from build123d import *

# Parameters (mm, degrees)
BOSS_EXTRUDE1_DEPTH = 80
SKETCH2_W           = 80
SKETCH2_H           = 80
BOSS_EXTRUDE2_DEPTH = 790


with BuildPart() as part:
    # Sketch1 → Boss-Extrude1 (new body)
    with BuildSketch(Plane.XY):
        Polygon((1040, 0), (0, 0), (0, -857.8), (80, -857.8), (80, -604.8), (960, -604.8), (960, -857.8), (1040, -857.8), align=None)
        Polygon((960, -524.8), (80, -524.8), (80, -361.670887123), (400.767069293, -80), (639.232930707, -80), (960, -361.670887123), align=None, mode=Mode.SUBTRACT)
        Polygon((729.892680056, -80), (960, -80), (960, -282.061056595), align=None, mode=Mode.SUBTRACT)
        Polygon((80, -282.061056595), (80, -80), (310.107319944, -80), align=None, mode=Mode.SUBTRACT)
    boss_extrude1 = extrude(amount=-BOSS_EXTRUDE1_DEPTH)

    # Sketch2 → Boss-Extrude2 (add)
    with BuildSketch(Plane(origin=(0, 0, -80), x_dir=(-1, 0, 0), z_dir=(0, 0, -1))):
        with Locations((-1000, -40)):
            Rectangle(SKETCH2_W, SKETCH2_H)
        with Locations((-40, -40)):
            Rectangle(SKETCH2_W, SKETCH2_H)
        with Locations((-520, -564.8)):
            Rectangle(SKETCH2_W, SKETCH2_H)
        with Locations((-520, -40)):
            Rectangle(SKETCH2_W, SKETCH2_H)
    boss_extrude2 = extrude(amount=BOSS_EXTRUDE2_DEPTH)

    # Mirror2: Boss-Extrude2 across plane
    add(boss_extrude2.mirror(Plane.XY.offset(-825)))

    # Mirror3: Boss-Extrude1 across plane
    add(boss_extrude1.mirror(Plane.XY.offset(-825)))


solid = part.part
The listing builds one solid part. Answer for the finished solid, in the listing's coordinates (mm). A direction names the side the tool comes from. Round coordinates to 2 decimals unless told otherwise and drop trailing zeros. Order: outer loops, then holes, each group sorted by start corner. A loop starts at its lowest first (then second) coordinate and runs counter-clockwise, first axis right, second up. Notation, with made-up numbers: M -22,38.5 L 4,38.5 A17 cw 4,54.5 Z; hole C 41.25,83 d6. An arc over 180 degrees is marked long. Answer in a Markdown table with one row per item. Add a question column.
1) The part is cut by section C-C on x = 179. Determine the outline of the cut face in (y, z), plus the area to 3 significant figures.
2) The part is cut by section B-B on y = -712. Determine the outline of the cut face in (x, z).
3) A flat-ended cylindrical pin translates along its axis: pin 1 Ø24 at (x, z) = (884.5, -38) entering from -Y. Find the tip coordinate at first contact, or state that the pin passes through.
4) The part is cut by section A-A on z = -1207. Determine the outline of the cut face in (x, y).
5) Consider line 1 along X through (y, z) = (-76.5, -1230); line 2 along Z through (x, y) = (420, -37.5); line 3 along Y through (x, z) = (486, -1261.5). Determine where each line is inside the solid, lowest interval first. Write a range as from..to.
6) The part is cut by section D-D on y = -104.5. Count the separate pieces of the cut face and the enclosed holes in it, plus the area to 3 significant figures.
7) Determine the mould class of faces 5 (the face through (1001, -80, -835)), 6 (the face through (960, -180, -39)), 7 (the face through (556, -554, -1650)) for opening direction Z: pulls with the +Z half, pulls with the -Z half, needs draft (parallel to the pull), parting line crosses it, or undercut.
8) Which of the six approach directions +Z, -Z, +X, -X, +Y, -Y give full straight-line access (tool end or side, diameter ignored) to faces 1 (the face through (960, -41, -835)), 2 (the face through (960, -442, -1611)), 3 (the face through (80, -733, -1611)), 4 (the face through (132, -300, -80))?
Findings below:
| question | item | result |
|---|---|---|
| 1 | outline | M -604.8,-1650 L -524.8,-1650 L -524.8,-1570 L -604.8,-1570 Z; M -604.8,-80 L -524.8,-80 L -524.8,0 L -604.8,0 Z; M -274.74,-1650 L -195.13,-1650 L -195.13,-1570 L -274.74,-1570 Z; M -274.74,-80 L -195.13,-80 L -195.13,0 L -274.74,0 Z; M -80,-1650 L 0,-1650 L 0,-1570 L -80,-1570 Z; M -80,-80 L 0,-80 L 0,0 L -80,0 Z |
| 1 | area | 38,300 mm² |
| 2 | outline | M 0,-1650 L 80,-1650 L 80,-1570 L 0,-1570 Z; M 0,-80 L 80,-80 L 80,0 L 0,0 Z; M 960,-1650 L 1040,-1650 L 1040,-1570 L 960,-1570 Z; M 960,-80 L 1040,-80 L 1040,0 L 960,0 Z |
| 3 | pin 1 | stops at y = -604.8 |
| 4 | outline | M 0,-80 L 80,-80 L 80,0 L 0,0 Z; M 480,-604.8 L 560,-604.8 L 560,-524.8 L 480,-524.8 Z; M 480,-80 L 560,-80 L 560,0 L 480,0 Z; M 960,-80 L 1040,-80 L 1040,0 L 960,0 Z |
| 5 | line 1 | x = 0..80, 480..560, 960..1040 |
| 5 | line 2 | z = -1650..-1570, -80..0 |
| 5 | line 3 | y = -604.8..-524.8, -80..0 |
| 6 | separate pieces | 8 |
| 6 | enclosed holes | 0 |
| 6 | area | 54,600 mm² |
| 7 | face 5 | undercut |
| 7 | face 6 | needs draft |
| 7 | face 7 | pulls with the -Z half |
| 8 | face 1 | +Y, -Y |
| 8 | face 2 | +Z, -Z |
| 8 | face 3 | +Z, -Z, -Y |
| 8 | face 4 | -Y |
